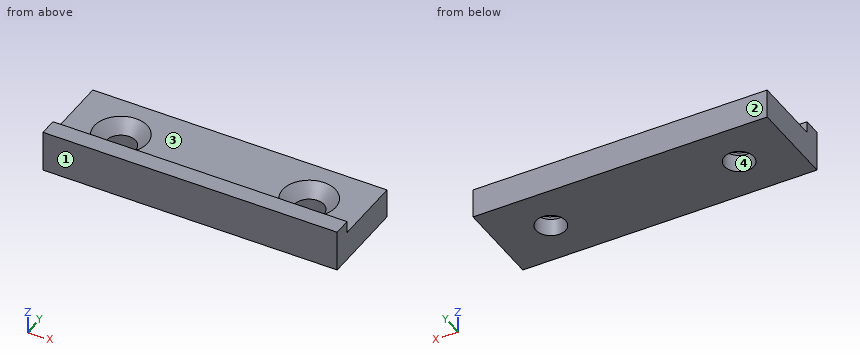
from build123d import *

# Parameters (mm, degrees)
F1_DEPTH       = 50
F3_D           = 5
F3_CSINK_D     = 9
F3_CSINK_ANGLE = 90


with BuildPart() as f1:
    # F0 (on Right) → F1 (new body)
    with BuildSketch(Plane.YZ):
        Polygon((-15, 0), (0, 0), (0, 5), (-12, 5), (-12, 7), (-15, 7), (-15, 5), align=None)
    extrude(amount=F1_DEPTH)

    # F3 (through all)
    with Locations(Plane.XY.offset(5)):
        with Locations((41, -7.5), (9, -7.5)):
            CounterSinkHole(F3_D / 2, F3_CSINK_D / 2, counter_sink_angle=F3_CSINK_ANGLE)


solid = f1.part
Could you check a few things on this model? Use its own coordinates, in mm. Face numbers are marked on the shaded views. Give positions to 0.01 mm unless a question says otherwise; leave off trailing zeros. Order: outer loops, then holes, each group sorted by start corner. A loop starts at its lowest first (then second) coordinate and runs counter-clockwise, first axis right, second up.
1. I need wall thicknesses on L1, parallel to X at y = -7.5, z = 1.35; L2, parallel to Y at x = 9, z = 1.7; L3, parallel to Z at x = 19, y = -8.75. Which ranges of each line are inside material? Lowest first, please.
Answers below:
L1: x = 0 to 6.5, 11.5 to 38.5, 43.5 to 50
L2: y = -15 to -10, -5 to 0
L3: z = 0 to 5
2. Suppose I cut it at D-D (z = 4). Write out the boundary of the cut face in (x, y), plus the area to 3 significant figures.
Answers below:
outline: (0, -15) - (50, -15) - (50, 0) - (0, 0) - close; hole circle Ø7 at (9, -7.5); hole circle Ø7 at (41, -7.5)
area: 673 mm2
3. Thinking about a two-plate mould opening in Y: for the marked faces 1, 2, 3 and 4, which applies, +Y half, -Y half, draft (parallel to the pull), parting line (faces both ways), or undercut?
Answers below:
face 1: -Y half
face 2: +Y half
face 3: draft
face 4: undercut
4. For pin 1 (4 mm diameter, centred on x = 36.5, y = -9, fed in from +Z); pin 2 (1 mm diameter, centred on x = 26.5, z = 1.5, fed in from +Y); pin 3 (1.6 mm diameter, centred on x = 24.5, z = 6, fed in from +Y); pin 4 (8 mm diameter, centred on x = 41, y = -7.5, fed in from +Z), each with a flat end and sliding along its axis, tell me the tip position at first contact or that it passes through.
Answers below:
pin 1: stops at z = 5
pin 2: stops at y = 0
pin 3: stops at y = -12
pin 4: stops at z = 4.5
5. Suppose I cut it at C-C (x = 26). Write out the boundary of the cut face in (y, z), plus the area to 3 significant figures.
Answers below:
outline: (-15, 0) - (0, 0) - (0, 5) - (-12, 5) - (-12, 7) - (-15, 7) - close
area: 81.0 mm2
6. Suppose I cut it at A-A (y = -7.5). Write out the boundary of the cut face in (x, z), plus the area to 3 significant figures.
Answers below:
outline: (0, 0) - (6.5, 0) - (6.5, 3) - (4.5, 5) - (0, 5) - close; (11.5, 0) - (38.5, 0) - (38.5, 3) - (36.5, 5) - (13.5, 5) - (11.5, 3) - close; (43.5, 0) - (50, 0) - (50, 5) - (45.5, 5) - (43.5, 3) - close
area: 192 mm2
7. Suppose I cut it at B-B (z = 0.75). Write out the boundary of the cut face in (x, y).
Answers below:
outline: (0, -15) - (50, -15) - (50, 0) - (0, 0) - close; hole circle Ø5 at (9, -7.5); hole circle Ø5 at (41, -7.5)
